from build123d import *

# Parameters (mm, degrees)
F0_R     = 3.175
F0_R_2   = 3.686252
F0_R_3   = 5.045636
F0_R_4   = 4.135696
F0_R_5   = 3.3448
F1_DEPTH = 25.4


with BuildPart() as f1:
    # F0 (on Front) → F1 (new body)
    with BuildSketch(Plane.XZ):
        with BuildLine():
            ThreePointArc((-52.450832, 60.008334), (-42.925832, 50.483334), (-33.400832, 60.008334))
            ThreePointArc((-33.400832, 60.008334), (-42.925832, 69.533334), (-52.450832, 60.008334))
        make_face()
        with Locations((-42.925832, 60.008334)):
            Circle(F0_R, mode=Mode.SUBTRACT)
        with BuildLine():
            Line((-27.178375, 11.216623), (-33.400832, 60.008334))
            ThreePointArc((-33.400832, 60.008334), (-42.925832, 50.483334), (-52.450832, 60.008334))
            Line((-52.450832, 60.008334), (-58.673289, 11.216623))
            ThreePointArc((-58.673289, 11.216623), (-42.925832, 25.083334), (-27.178375, 11.216623))
        make_face()
        with Locations((-48.560176, 45.733534)):
            Circle(F0_R_2, mode=Mode.SUBTRACT)
        with BuildLine():
            ThreePointArc((-27.050832, 9.208334), (-27.08275, 10.214501), (-27.178375, 11.216623))
            ThreePointArc((-27.178375, 11.216623), (-42.925832, 25.083334), (-58.673289, 11.216623))
            ThreePointArc((-58.673289, 11.216623), (-58.800832, 9.208334), (-58.673289, 7.200044))
            ThreePointArc((-58.673289, 7.200044), (-42.925832, -6.666666), (-27.178375, 7.200044))
            ThreePointArc((-27.178375, 7.200044), (-27.08275, 8.202166), (-27.050832, 9.208334))
        make_face()
        with Locations((-42.925832, 9.208334)):
            Circle(F0_R_3, mode=Mode.SUBTRACT)
        with BuildLine():
            ThreePointArc((-27.178375, 7.200044), (-42.925832, -6.666666), (-58.673289, 7.200044))
            Line((-58.673289, 7.200044), (-52.450832, -54.291666))
            ThreePointArc((-52.450832, -54.291666), (-42.925832, -44.766666), (-33.400832, -54.291666))
            ThreePointArc((-33.400832, -54.291666), (-35.954542, -60.782178), (-42.246341, -63.792399))
            Line((-42.246341, -63.792399), (1.524168, -62.229166))
            ThreePointArc((1.524168, -62.229166), (-6.412075, -54.150441), (1.806574, -46.359192))
            Line((1.806574, -46.359192), (-23.959184, -45.441901))
            ThreePointArc((-23.959184, -45.441901), (-29.666072, -42.724413), (-31.586747, -36.702426))
            Line((-31.586747, -36.702426), (-27.178375, 7.200044))
        make_face()
        with BuildLine():
            ThreePointArc((-33.400832, -54.291666), (-42.925832, -44.766666), (-52.450832, -54.291666))
            ThreePointArc((-52.450832, -54.291666), (-49.661024, -61.026858), (-42.925832, -63.816666))
            Line((-42.925832, -63.816666), (-42.246341, -63.792399))
            ThreePointArc((-42.246341, -63.792399), (-35.954542, -60.782178), (-33.400832, -54.291666))
        make_face()
        with Locations((-42.925832, -54.291666)):
            Circle(F0_R_4, mode=Mode.SUBTRACT)
        with BuildLine():
            Line((-42.246341, -63.792399), (-42.925832, -63.816666))
            ThreePointArc((-42.925832, -63.816666), (-42.58587, -63.810597), (-42.246341, -63.792399))
        make_face()
        with BuildLine():
            ThreePointArc((9.461668, -54.291666), (7.235801, -48.779756), (1.806574, -46.359192))
            ThreePointArc((1.806574, -46.359192), (-6.412075, -54.150441), (1.524168, -62.229166))
            ThreePointArc((1.524168, -62.229166), (7.136828, -59.904326), (9.461668, -54.291666))
        make_face()
        with Locations((1.524168, -54.291666)):
            Circle(F0_R_5, mode=Mode.SUBTRACT)
    extrude(amount=F1_DEPTH)


solid = f1.part
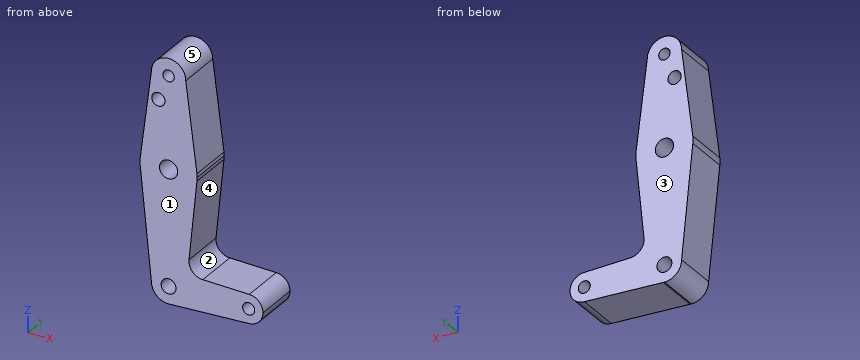
Read the model definition and answer for the solid it produces. Units are mm, in the model's axes. Face numbers are marked on the shaded views. A direction names the side the tool comes from. Round coordinates to 2 decimals unless told otherwise and drop trailing zeros. Write each loop counter-clockwise with the first axis right and the second up, starting at its lowest first coordinate (ties: lowest second). Pieces come first, ordered by that corner, then holes.
1. The part is cut by section A-A, the plane z = 44. Determine the outline of the cut face in (x, y), then the cut area to 3 significant figures.
2. Determine the mould class of the marked faces 1, 2 and 3 for opening direction Y: pulls with the +Y half, pulls with the -Y half, needs draft (parallel to the pull), parting line crosses it, or undercut.
3. The part is cut by section D-D, the plane z = -22.5. Determine the outline of the cut face in (x, y).
4. Straight lines are drawn through the part: L1, parallel to X at y = -18.75, z = -55.5; L2, parallel to Z at x = 3, y = -17; L3, parallel to Z at x = -50, y = -1.75. For each, find the intervals that lie inside material, in ascending order.
5. Which of the six approach directions +Z, -Z, +X, -X, +Y, -Y give full straight-line access (tool end or side, diameter ignored) to the marked faces 4 and 5?
6. Given pin 1 Ø1 at (x, y) = (-39, -4) entering from +Z; pin 2 Ø2 at (y, z) = (-10.5, 29.5) entering from -X; pin 3 Ø8 at (x, y) = (-28, -9.5) entering from -Z, each flat-ended and moving along its own axis, determine where each tip first touches the part or whether it passes through.
7. The part is cut by section C-C, the plane y = -4.5. State how many separate pieces and enclosed holes the cut face has, then the cut area to 3 significant figures.
8. The part is cut by section B-B, the plane x = -30. Determine the outline of the cut face in (y, z), then the cut area to 3 significant figures.
Values:
1. outline: (-54.49, -25.4) - (-51.81, -25.4) - (-51.81, 0) - (-54.49, 0) - close; (-45.31, -25.4) - (-31.36, -25.4) - (-31.36, 0) - (-45.31, 0) - close
1. area: 422 mm2
2. face 1: pulls with the -Y half
2. face 2: needs draft
2. face 3: pulls with the +Y half
3. outline: (-55.67, -25.4) - (-30.16, -25.4) - (-30.16, 0) - (-55.67, 0) - close
4. L1: x = -52.37 to -46.88, -38.97 to -1.59, 4.64 to 9.37
4. L2: z = -62.09 to -57.29, -51.29 to -46.49
4. L3: z = -60.67 to 42.34, 49.13 to 66.39
5. face 4: +X, +Y, -Y
5. face 5: +Z, +Y, -Y
6. pin 1: stops at z = 68.9
6. pin 2: stops at x = -56.47
6. pin 3: stops at z = -63.43
7. separate pieces: 1
7. enclosed holes: 5
7. area: 3,680 mm2
8. outline: (-25.4, -63.36) - (0, -63.36) - (0, -42.32) - (-25.4, -42.32) - close; (-25.4, -20.9) - (0, -20.9) - (0, 33.34) - (-25.4, 33.34) - close
8. area: 1,910 mm2
